For this review, use the dimensioned drawing (mm, ordinates from the lowest corner) and the shaded views. A direction names the side the tool comes from. Give positions to 0.01 mm unless a question says otherwise; leave off trailing zeros. Order: outer loops, then holes, each group sorted by start corner. A loop starts at its lowest first (then second) coordinate and runs counter-clockwise, first axis right, second up. Notation, with made-up numbers: (2.5, -18) -> (22.5, -18) arc R34 cw to (22.5, 20) -> close; hole circle Ø7 at (36, 68). An arc over 180 degrees is marked (long way). Answer as a JSON object with one key per item and string values. Group by question number.
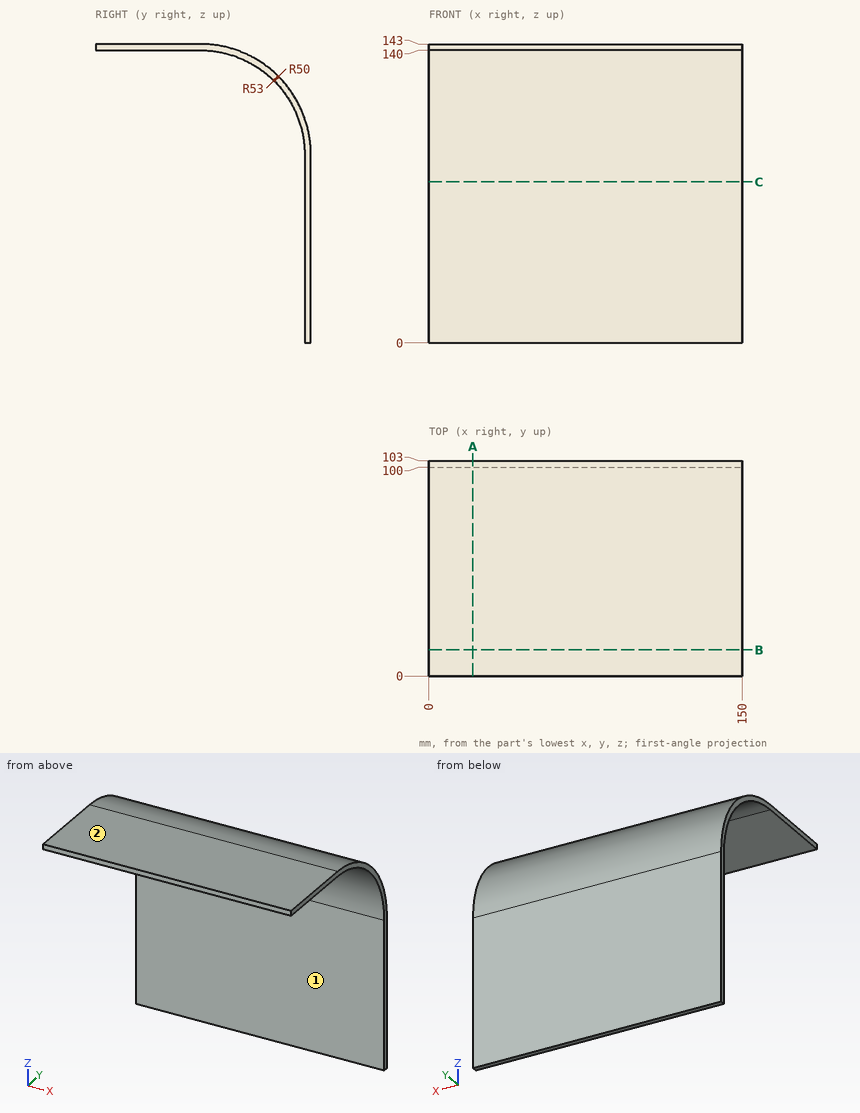
1. Machinability: for the marked faces 1 and 2, which of the approach directions +Z, -Z, +X, -X, +Y, -Y give a long, thin tool a straight path to every point of the face, cutting with its end or side? Answer none if there is none.
2. For pin 1 (12 mm diameter, centred on x = 84, y = 67.5, fed in from +Z); pin 2 (10 mm diameter, centred on x = 58, z = 39.5, fed in from -Y); pin 3 (4 mm diameter, centred on x = 104.5, y = 84, fed in from +Z), all flat-tipped, find the tip position at first contact; note any pin that passes through.
3. Take a section at C-C on z = 77. Give the boundary of the cut face in (x, y).
4. Take a section at A-A on x = 21. Give the boundary of the cut face in (y, z).
5. For probe 1 along Y at (x, z) = (108.5, 52); probe 2 along Z at (x, y) = (101.5, 36); probe 3 along Z at (x, y) = (124, 69.5), list the stretches that pass through material, from the lowest coordinate up. Write a range as [from, to].
6. Take a section at B-B on y = 12.5. Give the boundary of the cut face in (x, z).
Checks:
{
 "1": {"face 1": "-Z, +X, -X, -Y", "face 2": "+Z, +X, -X, +Y, -Y"},
 "2": {"pin 1": "stops at z = 141.74", "pin 2": "stops at y = 100", "pin 3": "stops at z = 132.25"},
 "3": {"outline": "(0, 100) -> (150, 100) -> (150, 103) -> (0, 103) -> close"},
 "4": {"outline": "(0, 140) -> (50, 140) arc R50 cw to (100, 90) -> (100, 0) -> (103, 0) -> (103, 90) arc R53 ccw to (50, 143) -> (0, 143) -> close"},
 "5": {"probe 1": "y = [100, 103]", "probe 2": "z = [140, 143]", "probe 3": "z = [136.04, 139.28]"},
 "6": {"outline": "(0, 140) -> (150, 140) -> (150, 143) -> (0, 143) -> close"}
}
